from build123d import *

# Parameters (mm, degrees)
SKETCH1_R           = 35
BOSS_EXTRUDE1_DEPTH = 12


with BuildPart() as part:
    # Sketch1 → Boss-Extrude1 (new body)
    with BuildSketch(Plane(origin=(0, 0, 0), x_dir=(0, 0, -1), z_dir=(1, 0, 0))):
        Circle(SKETCH1_R)
        with BuildLine():
            Line((-2.073644135, 1.65), (2.073644135, 1.65))
            ThreePointArc((2.073644135, 1.65), (2.65, 0), (2.073644135, -1.65))
            Line((2.073644135, -1.65), (-2.073644135, -1.65))
            ThreePointArc((-2.073644135, -1.65), (-2.65, 0), (-2.073644135, 1.65))
        make_face(mode=Mode.SUBTRACT)
    extrude(amount=-BOSS_EXTRUDE1_DEPTH)


solid = part.part
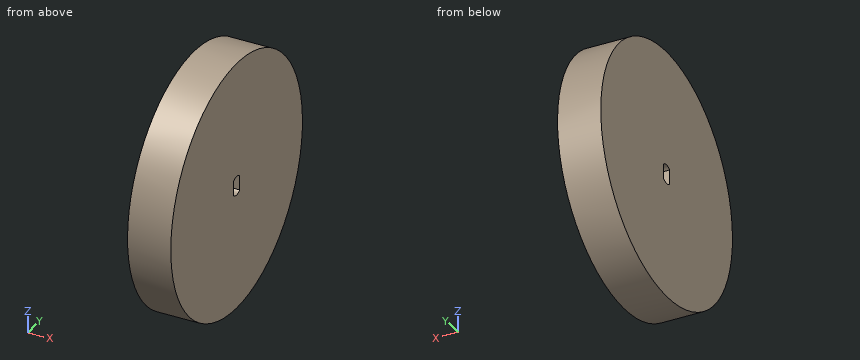
Can you work these out from the model? Positions are in its coordinate system, mm. Coordinates: 2 decimals unless noted, no trailing zeros. Loops run counter-clockwise (first coordinate to the right, second up) from the corner with the lowest first, then second, coordinate; pieces in that order, holes last. Notation, with made-up numbers: M 82,52.5 L 116,52.5 A16 ccw 116,68.5 Z; hole C 29.5,-33 d5. An arc over 180 degrees is marked long. Return JSON: item names as keys, results as strings. Group by question number.
Item 1: If I drill on L1, parallel to Y at x = -6.5, z = 0; L2, parallel to Z at x = -3.5, y = 1; L3, parallel to Z at x = -10, y = -11.5, over which ranges is the centre line in solid material (lowest first)? Write a range as from..to.
Item 2: Imagine slicing it at B-B (z = 0). Please give me the cut outline in (x, y), and give its area (3 significant figures).
Item 3: Imagine slicing it at A-A (y = 0). Please give me the cut outline in (x, z), and give its area (3 significant figures).
Item 4: I'm going to push flat-ended pins straight in: pin 1 Ø4.5 at (x, z) = (-9, -0.5) entering from +Y; pin 2 Ø2 at (x, z) = (-5.5, -6) entering from +Y; pin 3 Ø6 at (y, z) = (-11, 11.5) entering from +X; pin 4 Ø5 at (x, y) = (-6.5, 21) entering from +Z. Where does each tip first touch, or does it pass through?
Item 5: Imagine slicing it at C-C (x = -3.25). Please give me the cut outline in (y, z), and give its area (3 significant figures).
Item 6: Imagine slicing it at D-D (y = 28). Please give me the cut outline in (x, z), and give its area (3 significant figures).
Verdict:
{
 "1": {"L1": "y = -35..-1.65, 1.65..35", "L2": "z = -34.99..-2.45, 2.45..34.99", "L3": "z = -33.06..33.06"},
 "2": {"outline": "M -12,-35 L 0,-35 L 0,-1.65 L -12,-1.65 Z; M -12,1.65 L 0,1.65 L 0,35 L -12,35 Z", "area": "800 mm^2"},
 "3": {"outline": "M -12,-35 L 0,-35 L 0,-2.65 L -12,-2.65 Z; M -12,2.65 L 0,2.65 L 0,35 L -12,35 Z", "area": "776 mm^2"},
 "4": {"pin 1": "stops at y = 35", "pin 2": "stops at y = 34.64", "pin 3": "stops at x = 0", "pin 4": "stops at z = 29.71"},
 "5": {"outline": "C 0,0 d70; hole M -1.65,-2.07 A2.65 ccw 1.65,-2.07 L 1.65,2.07 A2.65 ccw -1.65,2.07 Z", "area": "3,830 mm^2"},
 "6": {"outline": "M -12,-21 L 0,-21 L 0,21 L -12,21 Z", "area": "504 mm^2"}
}
